Job drawing, mm, ordinate dimensions from the low corner. One solid piece. A direction names the side the tool comes from. Round coordinates to 2 decimals unless told otherwise and drop trailing zeros. Loops run counter-clockwise (first coordinate to the right, second up) from the corner with the lowest first, then second, coordinate; pieces in that order, holes last. Notation, with made-up numbers: M -28,89 L -4,89 A21 cw -4,97 Z; hole C 29,80.5 d8. An arc over 180 degrees is marked long. Use one line per item in the form item = value.
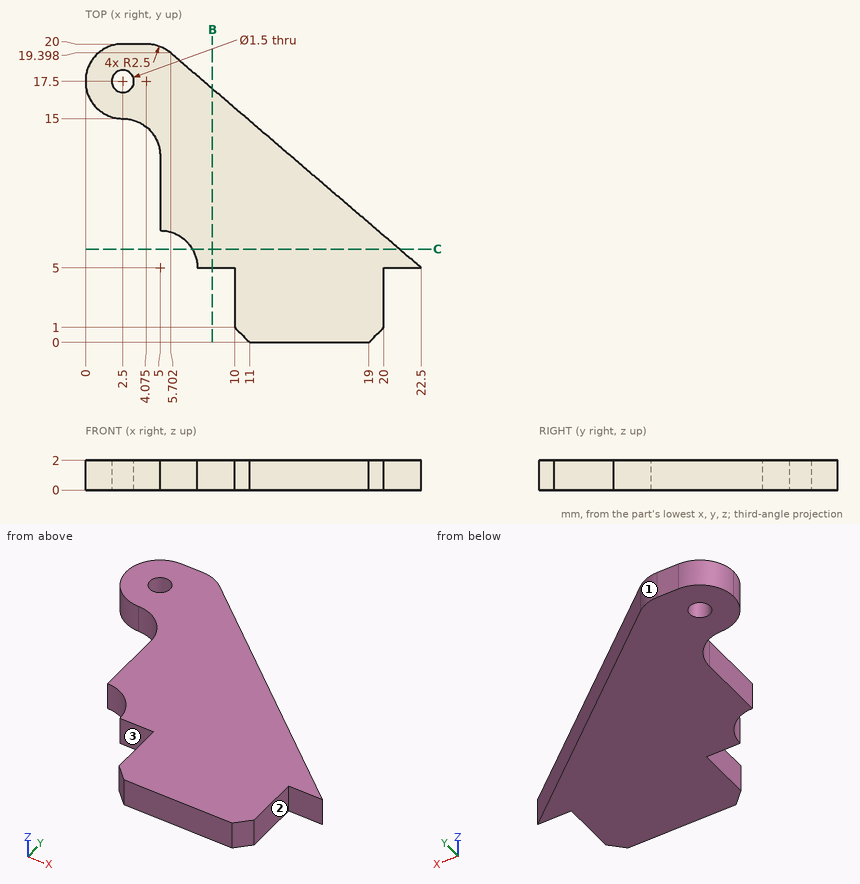
1. Cut at B-B on x = 8.5. Write the cut outline in (y, z), and give its area (3 significant figures).
Completed:
outline = M 5,0 L 17,0 L 17,2 L 5,2 Z
area = 24.0 mm2
2. Tool access for the marked faces 1, 2 and 3: list every direction of +Z, -Z, +X, -X, +Y, -Y with a clear straight run to the whole face (end or side of a thin tool).
Completed:
face_1 = +Z, -Z, +X, +Y
face_2 = +Z, -Z, +X, -Y
face_3 = +Z, -Z, -X, -Y
3. Drop flat-ended pins along their axis: P1, Ø0.6, axis at y = 10, z = 1, coming from the -X side; P2, Ø1, axis at y = 2.5, z = 1, coming from the -X side; P3, Ø1, axis at x = 10.5, z = 0.5, coming from the +Y side (1 decimal); P4, Ø0.9, axis at x = 2.5, y = 17.5, coming from the +Z side. Give the stop position or say it passes through.
Completed:
P1 = 5
P2 = 10
P3 = 15.7
P4 = through
4. Probe line 1 along Y through (x, z) = (2.5, 1.2); line 2 along X through (y, z) = (4.25, 0.95); line 3 along Y through (x, z) = (13.75, 1.45). List the from-to ranges inside material, lowest first. Write a range as from..to.
Completed:
line_1 = 15..16.75, 18.25..20
line_2 = 10..20
line_3 = 0..12.5
5. Cut at C-C on y = 6.25. Write the cut outline in (x, z) (1 decimal).
Completed:
outline = M 7.2,0 L 21,0 L 21,2 L 7.2,2 Z
